Verification items for the finished model (mm, model axes). A direction names the side the tool comes from. Coordinates: 2 decimals unless noted, no trailing zeros. Write each loop counter-clockwise with the first axis right and the second up, starting at its lowest first coordinate (ties: lowest second). Pieces come first, ordered by that corner, then holes. Notation, with made-up numbers: (62, -19.75) -> (100, -19.75) arc R18 ccw to (100, -0.75) -> close; hole circle Ø3 at (41.5, 2.25). An arc over 180 degrees is marked (long way). Write item = value, one per line. Start each with the question number.
(1) Gauge pin test, flat ends, axial feed: pin 1 Ø2.5 at (x, y) = (34.5, -0.5) entering from +Z; pin 2 Ø2 at (y, z) = (-0.5, 11.5) entering from -X; pin 3 Ø1.5 at (x, y) = (4.5, -1) entering from +Z; pin 4 Ø6.5 at (x, z) = (0, 45) entering from +Y. Record the tip position at first contact, or that the pin passes through.
(2) Section check C-C (x = 19). Record the cut outline in (y, z).
(3) Material ranges on probe 1 along Z at (x, y) = (45, 0.9); probe 2 along X at (y, z) = (-0.85, 45); probe 3 along Z at (x, y) = (32.5, 0.8), recorded low to high. Write a range as [from, to].
(4) Section check D-D (z = 12.5). Record the cut outline in (x, y).
(5) Section check A-A (z = 1). Record the cut outline in (x, y).
(6) Mould release check, pull along X, two halves, no side actions. Record for faces 1 (the face through (30, 1, 8)), 2 (the face through (-0.867, -1.232, -3.905)), 3 (the face through (25.47, -0.25, -0.11)): released by +X, released by -X, zero draft, split by the parting line, or undercut.
(7) Set-up check for faces 4 (the face through (3, 0, 24)), 5 (the face through (40, 0, 0)), 6 (the face through (3, -2.5, 25)), 7 (the face through (10.627, -1.268, 29.552)): record each of +Z, -Z, +X, -X, +Y, -Y from which the full face is reachable in a straight line by a thin tool's end or side.
(8) Section check B-B (z = 47). Record the cut outline in (x, y), plus the area to 3 significant figures.
```python
from build123d import *

# Parameters (mm, degrees)
F0_R     = 4
F0_R_2   = 3
F1_DEPTH = 2.5
F2_W     = 12
F2_H     = 2.5
F2_W_2   = 8
F3_DEPTH = 65.001


with BuildPart() as f1:
    # F0 (on Front) → F1 (new body, symmetric)
    with BuildSketch(Plane.XZ):
        with BuildLine():
            ThreePointArc((45, -8), (53, 0), (45, 8))
            Line((45, 8), (15.268102, 8))
            ThreePointArc((15.268102, 8), (10.841623, 9.949533), (9.291666, 14.531239))
            Line((9.291666, 14.531239), (12, 45))
            ThreePointArc((12, 45), (0, 57), (-12, 45))
            Line((-12, 45), (-8, 0))
            ThreePointArc((-8, 0), (-5.656854, -5.656854), (0, -8))
            Line((0, -8), (45, -8))
        make_face()
        Circle(F0_R, mode=Mode.SUBTRACT)
        with Locations((45, 0)):
            Circle(F0_R_2, mode=Mode.SUBTRACT)
        with Locations((0, 45)):
            Circle(F0_R, mode=Mode.SUBTRACT)
    extrude(amount=F1_DEPTH, both=True)

    # F2 (on face) → F3 (cut, through all)
    with BuildSketch(Plane(origin=(0, 0, -8), x_dir=(1, 0, 0), z_dir=(0, 0, -1))):
        with Locations((-6, -1.25)):
            Rectangle(F2_W, F2_H)
        with BuildLine():
            Line((17.572512, 0), (0, 0))
            Line((0, 0), (0, -2.5))
            Line((0, -2.5), (27.427488, -2.5))
            ThreePointArc((27.427488, -2.5), (24.885705, -2.182628), (22.5, -1.25))
            ThreePointArc((22.5, -1.25), (20.114295, -0.317372), (17.572512, 0))
        make_face()
        with Locations((49, 1.25)):
            Rectangle(F2_W_2, F2_H)
        with BuildLine():
            Line((45, 2.5), (17.572512, 2.5))
            ThreePointArc((17.572512, 2.5), (20.729021, 2.105872), (23.691705, 0.94769))
            ThreePointArc((23.691705, 0.94769), (25.500431, 0.240616), (27.427488, 0))
            Line((27.427488, 0), (45, 0))
            Line((45, 0), (45, 2.5))
        make_face()
    extrude(amount=-F3_DEPTH, mode=Mode.SUBTRACT)


solid = f1.part
```
Response:
q1.pin_1 = 8
q1.pin_2 = -9.11
q1.pin_3 = 56.4
q1.pin_4 = through
q2.outline = (-2.42, -8) -> (0.1, -8) -> (0.1, 8) -> (-2.42, 8) -> close
q3.probe_1 = [-8, -3], [3, 8]
q3.probe_2 = [-12, -4], [4, 12]
q3.probe_3 = [-8, 8]
q4.outline = (-9.11, -2.5) -> (9.46, -2.5) -> (9.46, 0) -> (-9.11, 0) -> close
q5.outline = (-8.09, -2.5) -> (-3.87, -2.5) -> (-3.87, 0) -> (-8.09, 0) -> close; (3.87, -2.5) -> (17.57, -2.5) arc R12.84 ccw to (23.69, -0.95) arc R7.84 cw to (27.43, 0) -> (42.17, 0) -> (42.17, 2.5) -> (27.43, 2.5) arc R10.34 ccw to (22.5, 1.25) arc R10.34 cw to (17.57, 0) -> (3.87, 0) -> close; (47.83, 0) -> (52.94, 0) -> (52.94, 2.5) -> (47.83, 2.5) -> close
q6.face_1 = zero draft
q6.face_2 = undercut
q6.face_3 = released by +X
q7.face_4 = +Z, -Z, -X, +Y
q7.face_5 = +Z, -Z, +X, -Y
q7.face_6 = +Z, -Z, +X, -X, -Y
q7.face_7 = +X, +Y, -Y
q8.outline = (-11.83, -2.5) -> (-3.46, -2.5) -> (-3.46, 0) -> (-11.83, 0) -> close; (3.46, -2.5) -> (11.83, -2.5) -> (11.83, 0) -> (3.46, 0) -> close
q8.area = 41.8 mm2
